Here's how the part is built. I have some questions about the finished solid (model axes, mm). Face numbers are marked on the shaded views. A direction names the side the tool comes from. Round coordinates to 2 decimals unless told otherwise and drop trailing zeros. Write each loop counter-clockwise with the first axis right and the second up, starting at its lowest first coordinate (ties: lowest second). Pieces come first, ordered by that corner, then holes. Notation, with made-up numbers: (-27, 86.25) -> (-13, 86.25) arc R24 cw to (-13, 122.25) -> close; hole circle Ø10 at (61, -4.5). An arc over 180 degrees is marked (long way). Answer in a Markdown table with one row per item.
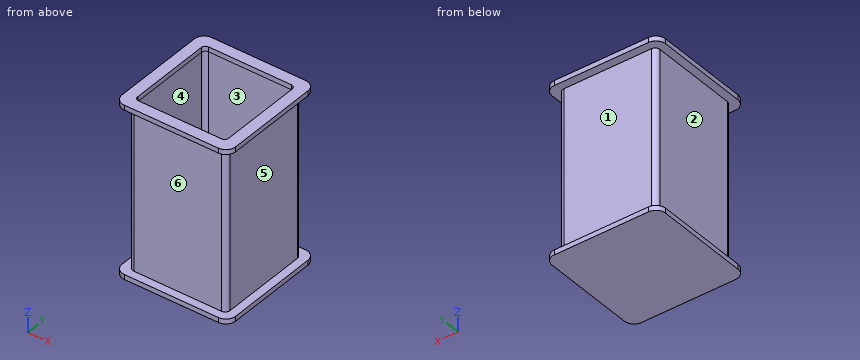
from build123d import *

# Parameters (mm, degrees)
BOSS_EXTRUDE1_DEPTH = 3
BOSS_EXTRUDE2_DEPTH = 100
BOSS_EXTRUDE3_DEPTH = 3


with BuildPart() as part:
    # Sketch1 → Boss-Extrude1 (new body)
    with BuildSketch(Plane(origin=(0, 0, 0), x_dir=(0, 1, 0), z_dir=(0, 0, 1))):
        with BuildLine():
            Line((-1, 63), (57, 63))
            ThreePointArc((57, 63), (61.242640687, 61.242640687), (63, 57))
            Line((63, 57), (63, -1))
            ThreePointArc((63, -1), (61.242640687, -5.242640687), (57, -7))
            Line((57, -7), (-1, -7))
            ThreePointArc((-1, -7), (-5.242640687, -5.242640687), (-7, -1))
            Line((-7, -1), (-7, 57))
            ThreePointArc((-7, 57), (-5.242640687, 61.242640687), (-1, 63))
        make_face()
    extrude(amount=-BOSS_EXTRUDE1_DEPTH)

    # Sketch2 → Boss-Extrude2 (add)
    with BuildSketch(Plane.XY):
        with BuildLine():
            Line((-54.993031309, 57.991494042), (-0.993031309, 57.991494042))
            ThreePointArc((-0.993031309, 57.991494042), (1.128289034, 57.112814386), (2.006968691, 54.991494042))
            Line((2.006968691, 54.991494042), (2.006968691, 0.991494042))
            ThreePointArc((2.006968691, 0.991494042), (1.128289034, -1.129826302), (-0.993031309, -2.008505958))
            Line((-0.993031309, -2.008505958), (-54.993031309, -2.008505958))
            ThreePointArc((-54.993031309, -2.008505958), (-57.114351653, -1.129826302), (-57.993031309, 0.991494042))
            Line((-57.993031309, 0.991494042), (-57.993031309, 54.991494042))
            ThreePointArc((-57.993031309, 54.991494042), (-57.114351653, 57.112814386), (-54.993031309, 57.991494042))
        make_face()
        with BuildLine():
            Line((-55.993031309, 2.491494042), (-55.993031309, 53.491494042))
            ThreePointArc((-55.993031309, 53.491494042), (-55.260798262, 55.259260995), (-53.493031309, 55.991494042))
            Line((-53.493031309, 55.991494042), (-2.493031309, 55.991494042))
            ThreePointArc((-2.493031309, 55.991494042), (-0.725264356, 55.259260995), (0.006968691, 53.491494042))
            Line((0.006968691, 53.491494042), (0.006968691, 2.491494042))
            ThreePointArc((0.006968691, 2.491494042), (-0.725264356, 0.723727089), (-2.493031309, -0.008505958))
            Line((-2.493031309, -0.008505958), (-53.493031309, -0.008505958))
            ThreePointArc((-53.493031309, -0.008505958), (-55.260798262, 0.723727089), (-55.993031309, 2.491494042))
        make_face(mode=Mode.SUBTRACT)
    extrude(amount=BOSS_EXTRUDE2_DEPTH)

    # Sketch4 → Boss-Extrude3 (add)
    with BuildSketch(Plane.XY.offset(100)):
        with BuildLine():
            Line((-56.993104306, 62.991512558), (1.006895694, 62.991512558))
            ThreePointArc((1.006895694, 62.991512558), (5.249536381, 61.234153245), (7.006895694, 56.991512558))
            Line((7.006895694, 56.991512558), (7.006895694, -1.008487442))
            ThreePointArc((7.006895694, -1.008487442), (5.249536381, -5.251128129), (1.006895694, -7.008487442))
            Line((1.006895694, -7.008487442), (-56.993104306, -7.008487442))
            ThreePointArc((-56.993104306, -7.008487442), (-61.235744993, -5.251128129), (-62.993104306, -1.008487442))
            Line((-62.993104306, -1.008487442), (-62.993104306, 56.991512558))
            ThreePointArc((-62.993104306, 56.991512558), (-61.235744993, 61.234153245), (-56.993104306, 62.991512558))
        make_face()
        with BuildLine():
            Line((-55.993104306, 2.491512558), (-55.993104306, 53.491512558))
            ThreePointArc((-55.993104306, 53.491512558), (-55.260871259, 55.259279511), (-53.493104306, 55.991512558))
            Line((-53.493104306, 55.991512558), (-2.493104306, 55.991512558))
            ThreePointArc((-2.493104306, 55.991512558), (-0.725337353, 55.259279511), (0.006895694, 53.491512558))
            Line((0.006895694, 53.491512558), (0.006895694, 2.491512558))
            ThreePointArc((0.006895694, 2.491512558), (-0.725337353, 0.723745605), (-2.493104306, -0.008487442))
            Line((-2.493104306, -0.008487442), (-53.493104306, -0.008487442))
            ThreePointArc((-53.493104306, -0.008487442), (-55.260871259, 0.723745605), (-55.993104306, 2.491512558))
        make_face(mode=Mode.SUBTRACT)
    extrude(amount=BOSS_EXTRUDE3_DEPTH)


solid = part.part
1) Which directions (+Z, -Z, +X, -X, +Y, -Y) give clear straight access to the entire face, cutting with the end or side of a thin tool? Please do the marked faces 4, 5 and 6.
Response:
| item | result |
|---|---|
| face 4 | +Z |
| face 5 | +X, +Y, -Y |
| face 6 | +X, -X, -Y |
2) For pin 1 (12 mm diameter, centred on y = 24, z = 27, fed in from -X); pin 2 (10 mm diameter, centred on x = -7, y = 17, fed in from +Z); pin 3 (6 mm diameter, centred on x = -22, z = 30.5, fed in from -Y), each with a flat end and sliding along its axis, tell me the tip position at first contact or that it passes through.
Response:
| item | result |
|---|---|
| pin 1 | stops at x = -57.99 |
| pin 2 | stops at z = 0 |
| pin 3 | stops at y = -2.01 |
3) I need wall thicknesses on line 1 (X direction, y = 5, z = 31); line 2 (Y direction, x = -22.5, z = 62.5); line 3 (Z direction, x = -29.5, y = 8.5). Which ranges of each line are inside material? Lowest first, please. Write a range as [from, to].
Response:
| item | result |
|---|---|
| line 1 | x = [-57.99, -55.99], [0.01, 2.01] |
| line 2 | y = [-2.01, -0.01], [55.99, 57.99] |
| line 3 | z = [-3, 0] |
4) We'd pull the mould along X, two halves only. Please class the marked faces 1, 2 and 3: +X half, -X half, draft (parallel to the pull), parting line (faces both ways), or undercut.
Response:
| item | result |
|---|---|
| face 1 | draft |
| face 2 | -X half |
| face 3 | undercut |
5) I want a section at C-C, the plane z = 32. List the corners of the cut face in (x, y) for me, and give its area (3 significant figures).
Response:
| item | result |
|---|---|
| outline | (-57.99, 0.99) arc R3 ccw to (-54.99, -2.01) -> (-0.99, -2.01) arc R3 ccw to (2.01, 0.99) -> (2.01, 54.99) arc R3 ccw to (-0.99, 57.99) -> (-54.99, 57.99) arc R3 ccw to (-57.99, 54.99) -> close; hole (-55.99, 2.49) arc R2.5 ccw to (-53.49, -0.01) -> (-2.49, -0.01) arc R2.5 ccw to (0.01, 2.49) -> (0.01, 53.49) arc R2.5 ccw to (-2.49, 55.99) -> (-53.49, 55.99) arc R2.5 ccw to (-55.99, 53.49) -> close |
| area | 462 mm^2 |
